Source: three-view drawing plus pictorial views. Frame: mm from the lowest corner of the part. Round coordinates to 2 decimals unless told otherwise and drop trailing zeros. Loops run counter-clockwise (first coordinate to the right, second up) from the corner with the lowest first, then second, coordinate; pieces in that order, holes last. Notation, with made-up numbers: M -28,-29.75 L -19,-29.75 A28 ccw -19,-2.75 Z; hole C 31.5,68.5 d11. An arc over 180 degrees is marked long. Return JSON: item names as keys, results as strings. Group by question number.
1) Material intervals for line 1 (Z direction, x = 3.5, y = 0.45); line 2 (Z direction, x = 12, y = 1.35); line 3 (Z direction, x = 21.25, y = 2.15), sorted ascending. Write a range as from..to.
2) Contact query for flat-ended pins moving along their axis: P1, Ø0.7, axis at y = 0.5, z = 12, coming from the +X side; P2, Ø3.5, axis at x = 12, z = 12, coming from the -Y side; P3, Ø4, axis at x = 6.34, z = 17.66, coming from the +Y side; P4, Ø1.1, axis at x = 19.5, y = 0.5, coming from the -Z side. Output: stop coordinate, or through.
3) Section A-A (x = 12). Output: boundary loops of the cut face in (y, z).
4) Section B-B (z = 12). Output: boundary loops of the cut face in (x, y).
5) Section C-C (x = 19.5). Output: boundary loops of the cut face in (y, z).
6) Section D-D (x = 7.25). Output: boundary loops of the cut face in (y, z).
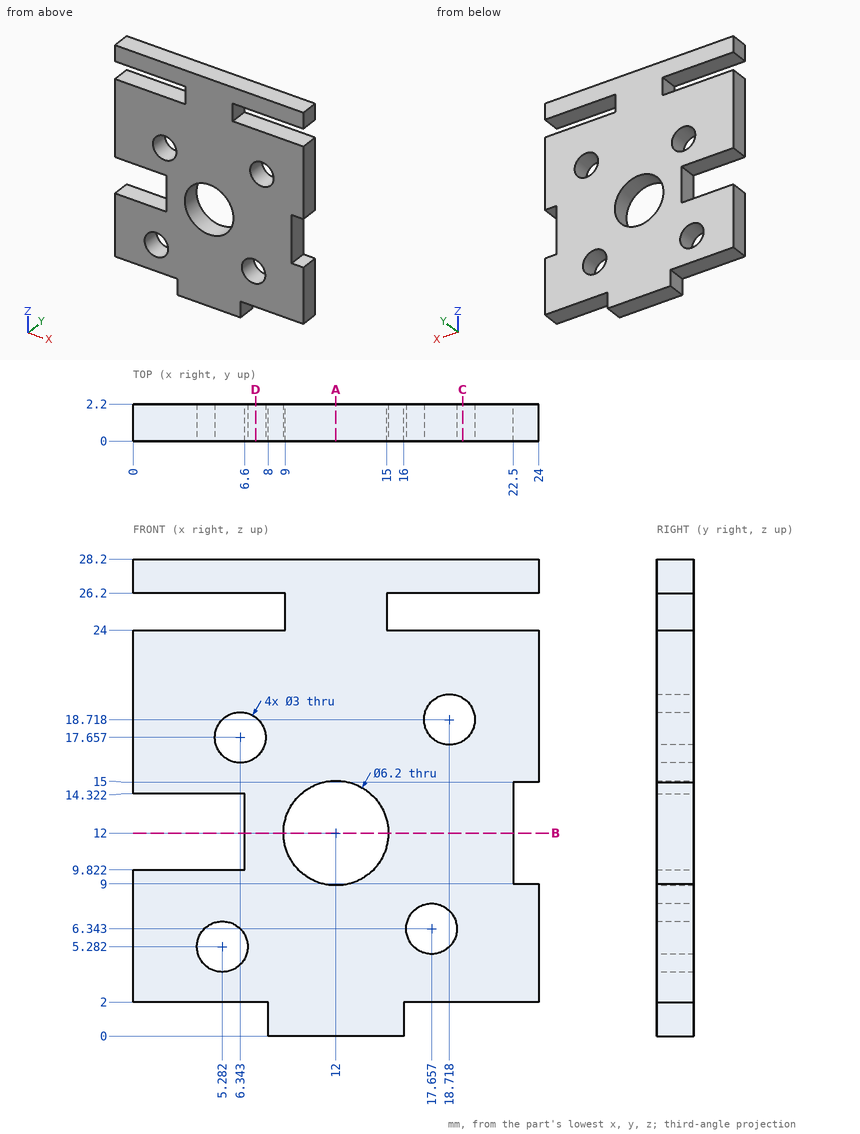
Returned:
{
 "1": {"line 1": "z = 2..9.82, 14.32..24, 26.2..28.2", "line 2": "z = 0..8.9, 15.1..28.2", "line 3": "z = 2..24, 26.2..28.2"},
 "2": {"P1": "stops at x = 22.5", "P2": "passes through", "P3": "stops at y = 2.2", "P4": "stops at z = 2"},
 "3": {"outline": "M 0,0 L 2.2,0 L 2.2,8.9 L 0,8.9 Z; M 0,15.1 L 2.2,15.1 L 2.2,28.2 L 0,28.2 Z"},
 "4": {"outline": "M 6.6,0 L 8.9,0 L 8.9,2.2 L 6.6,2.2 Z; M 15.1,0 L 22.5,0 L 22.5,2.2 L 15.1,2.2 Z"},
 "5": {"outline": "M 0,2 L 2.2,2 L 2.2,17.44 L 0,17.44 Z; M 0,20 L 2.2,20 L 2.2,24 L 0,24 Z; M 0,26.2 L 2.2,26.2 L 2.2,28.2 L 0,28.2 Z"},
 "6": {"outline": "M 0,2 L 2.2,2 L 2.2,16.46 L 0,16.46 Z; M 0,18.85 L 2.2,18.85 L 2.2,24 L 0,24 Z; M 0,26.2 L 2.2,26.2 L 2.2,28.2 L 0,28.2 Z"}
}
